Print and shaded views of the part. All mm, measured from the part's lowest x, y and z. A direction names the side the tool comes from. Give positions to 0.01 mm unless a question says otherwise; leave off trailing zeros. Loops run counter-clockwise (first coordinate to the right, second up) from the corner with the lowest first, then second, coordinate; pieces in that order, holes last.
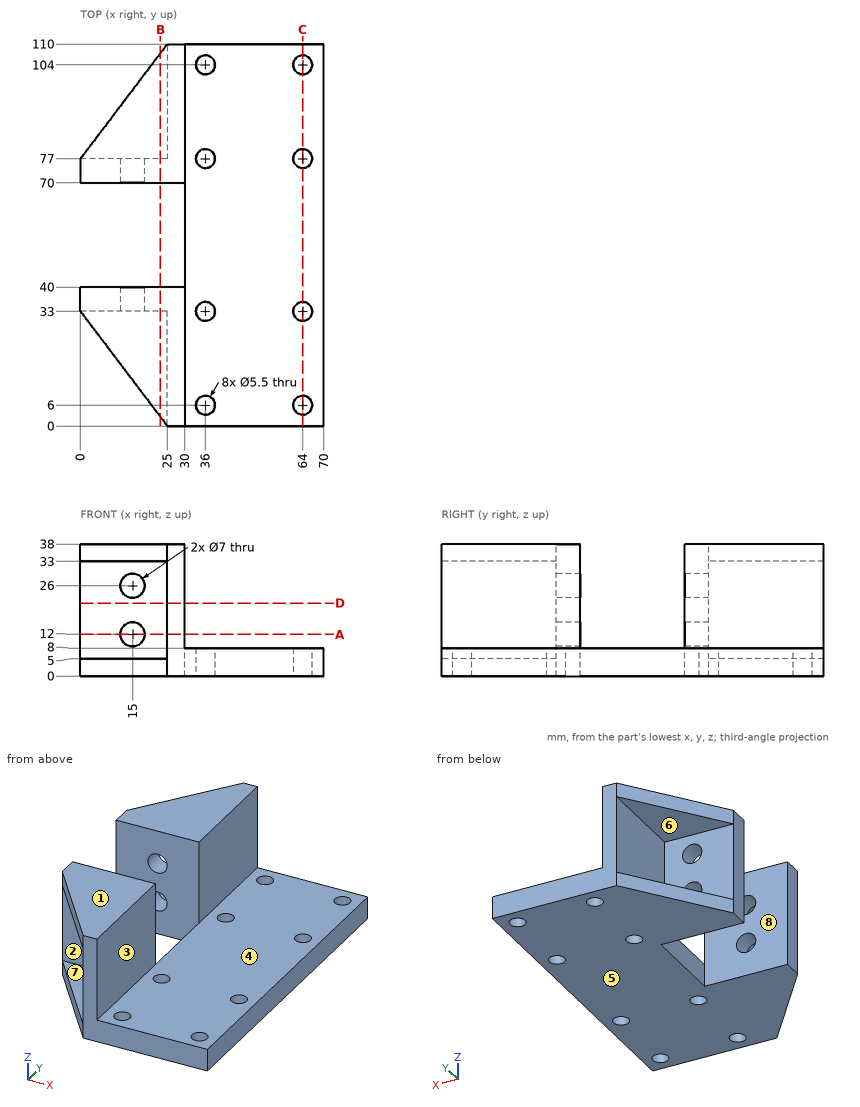
1. Saw through at D-D, the plane z = 21. List the corners of the cut face in (x, y), and give its area (3 significant figures).
Responses:
outline: (0, 33) - (25, 33) - (25, 0) - (30, 0) - (30, 40) - (0, 40) - close; (0, 70) - (30, 70) - (30, 110) - (25, 110) - (25, 77) - (0, 77) - close
area: 750 mm2
2. Saw through at C-C, the plane x = 64. List the corners of the cut face in (y, z).
Responses:
outline: (0, 0) - (3.25, 0) - (3.25, 8) - (0, 8) - close; (8.75, 0) - (30.25, 0) - (30.25, 8) - (8.75, 8) - close; (35.75, 0) - (74.25, 0) - (74.25, 8) - (35.75, 8) - close; (79.75, 0) - (101.25, 0) - (101.25, 8) - (79.75, 8) - close; (106.75, 0) - (110, 0) - (110, 8) - (106.75, 8) - close
3. Drop flat-ended pins along their axis: pin 1 (8 mm diameter, centred on x = 15, z = 12, fed in from -Y); pin 2 (14 mm diameter, centred on y = 20, z = 25.5, fed in from -X); pin 3 (9 mm diameter, centred on y = 57.5, z = 3.5, fed in from -X). Give the stop position or say it passes through.
Responses:
pin 1: stops at y = 33
pin 2: stops at x = 25
pin 3: stops at x = 30
4. Tool access for the marked faces 4, 5, 6, 7 and 8: list every direction of +Z, -Z, +X, -X, +Y, -Y with a clear straight run to the whole face (end or side of a thin tool).
Responses:
face 4: +Z, +X, +Y, -Y
face 5: -Z, +X, -X, +Y, -Y
face 6: -X, +Y
face 7: -X, -Y
face 8: +Z, -Z, -X
5. Saw through at A-A, the plane z = 12. List the corners of the cut face in (x, y), and give its area (3 significant figures).
Responses:
outline: (0, 33) - (11.5, 33) - (11.5, 40) - (0, 40) - close; (0, 70) - (11.5, 70) - (11.5, 77) - (0, 77) - close; (18.5, 33) - (25, 33) - (25, 0) - (30, 0) - (30, 40) - (18.5, 40) - close; (18.5, 70) - (30, 70) - (30, 110) - (25, 110) - (25, 77) - (18.5, 77) - close
area: 652 mm2
6. Saw through at B-B, the plane x = 23. List the corners of the cut face in (y, z), and give its area (3 significant figures).
Responses:
outline: (2.64, 0) - (40, 0) - (40, 38) - (2.64, 38) - (2.64, 33) - (33, 33) - (33, 5) - (2.64, 5) - close; (70, 0) - (107.36, 0) - (107.36, 5) - (77, 5) - (77, 33) - (107.36, 33) - (107.36, 38) - (70, 38) - close
area: 1,140 mm2
7. Probe line 1 along Y through (x, z) = (64, 3.75); line 2 along X through (y, z) = (33, 3); line 3 along Z through (x, y) = (15, 74.25). List the from-to ranges inside material, lowest first.
Responses:
line 1: y = 0 to 3.25, 8.75 to 30.25, 35.75 to 74.25, 79.75 to 101.25, 106.75 to 110
line 2: x = 0 to 33.25, 38.75 to 61.25, 66.75 to 70
line 3: z = 0 to 8.5, 15.5 to 22.5, 29.5 to 38
8. Pull direction Z, two halves, no side cores. Call the marked faces 1, 2 and 3: released by +Z, released by -Z, zero draft, split by the parting line, or undercut.
Responses:
face 1: released by +Z
face 2: undercut
face 3: zero draft
